Autodesk Inventor part; units mm, degrees
ref_plane "YZ Plane" through (0, 0, 0) normal (1, 0, 0) x (0, 1, 0)
ref_plane "XZ Plane" through (0, 0, 0) normal (0, 1, 0) x (-1, 0, 0)
ref_plane "XY Plane" through (0, 0, 0) normal (0, 0, 1) x (1, 0, 0)
sketch "Sketch1" plane through (0, 0, 0) normal (0, 0, 1) x (1, 0, 0)
  line L0 (0, 0) -> (14, 0)
  line L1 (14, 0) -> (14, -42)
  line L2 (14, -42) -> (0, -42)
  line L3 (0, -42) -> (0, 0)
  dimension "d0" = 14
  dimension "d1" = 42
extrude "Extrusion1" add sketch "Sketch1" along normal blind 6
sketch "Sketch2" plane through (14, -42, 0) normal (1, 0, 0) x (0, 0, -1)
  line L0 (-6, 30) -> (-27, 30)
  line L1 (-27, 30) -> (-27, 12)
  line L2 (-27, 12) -> (-6, 12)
  line L3 (-6, 12) -> (-6, 30)
  point P0 (0, 42)
  point P1 (-6, 0)
  point P2 (-6, 42)
extrude "Extrusion2" add sketch "Sketch2" against normal blind 14
sketch "Sketch3" plane through (14, -42, 0) normal (1, 0, 0) x (0, 0, -1)
  line L0 (0, 42) -> (0, 0)
  line L1 (-27, 30) -> (-6, 30)
  circle A0 centre (-17, 21) radius 4
  dimension "d11" = 8
extrude "Extrusion3" cut sketch "Sketch3" against normal blind 14
sketch "Sketch4" plane through (14, -42, 0) normal (1, 0, 0) x (0, 0, -1)
  point P0 (0, 42)
sketch "Sketch5" plane through (14, -42, 0) normal (1, 0, 0) x (0, 0, -1)
  point P0 (0, 42)
sketch "Sketch6" plane through (0, 0, 0) normal (0, 0, -1) x (-1, 0, 0)
  line L0 (0, -42) -> (-14, -42)
  circle A0 centre (-7, -5) radius 2.75
  circle A1 centre (-7, -37) radius 2.75
  point P0 (-14, 0)
  dimension "d16" = 5.5
  dimension "d17" = 5.5
extrude "Extrusion4" cut sketch "Sketch6" against normal blind 6
sketch "Sketch7" plane through (14, -42, 0) normal (1, 0, 0) x (0, 0, -1)
  point P0 (0, 42)
sketch "Sketch8" plane through (14, -42, 0) normal (1, 0, 0) x (0, 0, -1)
  line L0 (-27, 30) -> (-27, 12)
  line L1 (-27, 21) -> (-27, 22)
  line L2 (-27, 21) -> (-27, 20)
  line L3 (-27, 20) -> (-20.908, 20)
  line L4 (-27, 22) -> (-20.908, 22)
  line L5 (-20.908, 22) -> (-20.908, 20)
  point P0 (0, 42)
  dimension "d21" = 1
extrude "Extrusion5" cut sketch "Sketch8" against normal blind 14
sketch "Sketch9" plane through (14, -12, 27) normal (0, 1, 0) x (1, 0, 0)
  line L0 (0, 0) -> (-14, 0)
  line L1 (0, 21) -> (-14, 21)
  line L2 (-14, 0) -> (-14, 6.092)
  circle A0 centre (-7, 3.4183) radius 2.5
  point P0 (-14, 27)
  dimension "d24" = 5
extrude "Extrusion6" cut sketch "Sketch9" against normal blind 20
fillet "Fillet1" radius 2 1 edges at (7, -12, 6)
fillet "Fillet2" radius 2 1 edges at (7, -30, 6)
properties part number "soporte de eje de carril"
Check sheet for the modelled part. Datum: model origin and axes. Units: mm. A direction names the side the tool comes from. Give positions to 0.01 mm unless a question says otherwise; leave off trailing zeros. Loops run counter-clockwise (first coordinate to the right, second up) from the corner with the lowest first, then second, coordinate; pieces in that order, holes last. Notation, with made-up numbers: M 23.25,28.25 L 68.25,28.25 A17 cw 68.25,54.25 Z; hole C 44,-17.5 d6. An arc over 180 degrees is marked long. Return JSON: item names as keys, results as strings. Group by question number.
1. Cross-section at A-A on z = 17. Record the boundary of the cut face in (x, y), plus the area to 3 significant figures.
2. Mould release check, pull along Y, two halves, no side actions. Record for faces 1 (the cylindrical face through (5.73, -7.44, 2.96)), 2 (the flat face through (5.5, -20, 26)), 3 (the flat face through (7, 0, 3)), 4 (the cylindrical face through (6.9, -30.57, 6.6)): released by +Y, released by -Y, zero draft, split by the parting line, or undercut.
3. Tool access check on faces 5 (the flat face through (7, -26, 27)), 6 (the flat face through (7, -30, 18)), 7 (the flat face through (5.5, -22, 26)), 8 (the flat face through (4, -5, 6)). Record the directions out of +Z, -Z, +X, -X, +Y, -Y that give a thin tool (end or side, any length) a straight path to the whole face; none if there is none.
4. Cross-section at D-D on z = 22.75. Record the boundary of the cut face in (x, y), plus the area to 3 significant figures.
5. Cross-section at B-B on x = 7. State how many separate pieces and enclosed holes the cut face has, plus the area to 3 significant figures.
6. Cross-section at C-C on y = -5. Record the boundary of the cut face in (x, z).
7. Thickness scan on L1, parallel to Y at x = 7, z = 4.55; L2, parallel to Z at x = 7, y = -14; L3, parallel to Y at x = 8.5, z = 17.25. Record the ranges inside material, lowest first.
8. Go/stop test with flat-tipped pins: pin 1 (3 mm diameter, centred on x = 9.5, z = 24.5, fed in from +Y); pin 2 (5 mm diameter, centred on x = 5.5, z = 25.5, fed in from -Y); pin 3 (5 mm diameter, centred on x = 7, y = -4.5, fed in from +Z). Record where each tip stops, or that it passes through.
Return value:
{
 "1": {"outline": "M 0,-30 L 14,-30 L 14,-25 L 0,-25 Z; M 0,-17 L 14,-17 L 14,-12 L 0,-12 Z", "area": "140 mm^2"},
 "2": {"face 1": "undercut", "face 2": "undercut", "face 3": "released by +Y", "face 4": "released by -Y"},
 "3": {"face 5": "+Z, +X, -X, +Y, -Y", "face 6": "+Z, +X, -X, -Y", "face 7": "+Z, +X, -X", "face 8": "+Z, +X, -X, +Y"},
 "4": {"outline": "M 0,-30 L 4.64,-30 L 4.64,-22 L 0,-22 Z; M 0,-20 L 4.64,-20 L 4.64,-12 L 0,-12 Z; M 9.36,-30 L 14,-30 L 14,-22 L 9.36,-22 Z; M 9.36,-20 L 14,-20 L 14,-12 L 9.36,-12 Z", "area": "149 mm^2"},
 "5": {"separate pieces": "5", "enclosed holes": "0", "area": "423 mm^2"},
 "6": {"outline": "M 0,0 L 4.25,0 L 4.25,6 L 0,6 Z; M 9.75,0 L 14,0 L 14,6 L 9.75,6 Z"},
 "7": {"L1": "-42 to -39.75, -34.25 to -7.75, -2.25 to 0", "L2": "0 to 21.08, 26.08 to 27", "L3": "-30 to -24.99, -17.01 to -12"},
 "8": {"pin 1": "y = -12", "pin 2": "y = -30", "pin 3": "z = 6"}
}
